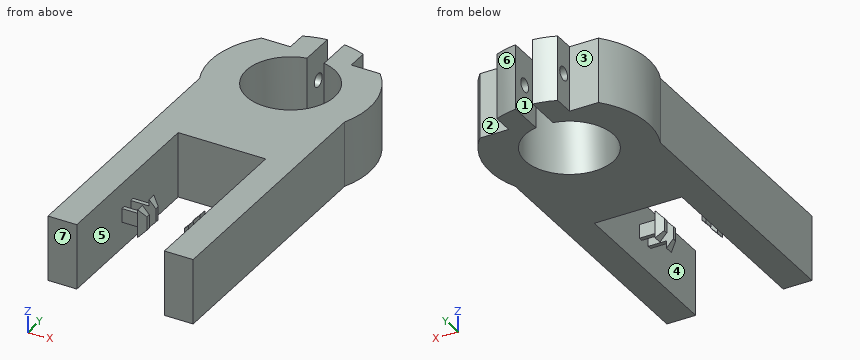
from build123d import *

# Parameters (mm, degrees)
F1_DEPTH = 41.91
F3_DEPTH = 132.842
F4_R     = 4.349558
F5_DEPTH = 93


with BuildPart() as f1:
    # F0 (on Top) → F1 (new body)
    with BuildSketch(Plane.XY):
        with BuildLine():
            ThreePointArc((5.462832, 27.789144), (0, -28.321), (-5.462832, 27.789144))
            Line((-5.462832, 27.789144), (-5.462832, 50.50542))
            ThreePointArc((-5.462832, 50.50542), (-12.596589, 49.213473), (-19.473793, 46.919201))
            Line((-19.473793, 46.919201), (-19.473793, 33.741264))
            Line((-19.473793, 33.741264), (-37.975875, 33.741264))
            ThreePointArc((-37.975875, 33.741264), (-50.191445, 7.839567), (-46.456356, -20.553516))
            Line((-46.456356, -20.553516), (-46.456356, -189.292356))
            Line((-46.456356, -189.292356), (-28.022196, -189.292356))
            Line((-28.022196, -189.292356), (-28.022196, -139.108405))
            Line((-28.022196, -139.108405), (-16.363064, -139.108405))
            Line((-16.363064, -139.108405), (-16.363064, -141.895995))
            Line((-16.363064, -141.895995), (-11.980078, -139.198765))
            Line((-11.980078, -139.198765), (-11.980078, -136.501536))
            Line((-11.980078, -136.501536), (-16.363064, -136.501536))
            Line((-16.363064, -136.501536), (-28.022196, -136.501536))
            Line((-28.022196, -136.501536), (-28.022196, -129.22018))
            Line((-28.022196, -129.22018), (-16.363064, -129.22018))
            Line((-16.363064, -129.22018), (-11.980078, -129.22018))
            Line((-11.980078, -129.22018), (-11.980078, -126.522951))
            Line((-11.980078, -126.522951), (-16.363064, -123.825721))
            Line((-16.363064, -123.825721), (-16.363064, -126.613311))
            Line((-16.363064, -126.613311), (-28.022196, -126.613311))
            Line((-28.022196, -126.613311), (-28.022196, -76.42936))
            Line((-28.022196, -76.42936), (0, -76.42936))
            Line((0, -76.42936), (28.022196, -76.42936))
            Line((28.022196, -76.42936), (28.022196, -126.613311))
            Line((28.022196, -126.613311), (16.363064, -126.613311))
            Line((16.363064, -126.613311), (16.363064, -123.825721))
            Line((16.363064, -123.825721), (11.980078, -126.522951))
            Line((11.980078, -126.522951), (11.980078, -129.22018))
            Line((11.980078, -129.22018), (16.363064, -129.22018))
            Line((16.363064, -129.22018), (28.022196, -129.22018))
            Line((28.022196, -129.22018), (28.022196, -136.501536))
            Line((28.022196, -136.501536), (16.363064, -136.501536))
            Line((16.363064, -136.501536), (11.980078, -136.501536))
            Line((11.980078, -136.501536), (11.980078, -139.198765))
            Line((11.980078, -139.198765), (16.363064, -141.895995))
            Line((16.363064, -141.895995), (16.363064, -139.108405))
            Line((16.363064, -139.108405), (28.022196, -139.108405))
            Line((28.022196, -139.108405), (28.022196, -189.292356))
            Line((28.022196, -189.292356), (46.456356, -189.292356))
            Line((46.456356, -189.292356), (46.456356, -20.553516))
            ThreePointArc((46.456356, -20.553516), (50.191445, 7.839567), (37.975875, 33.741264))
            Line((37.975875, 33.741264), (19.473793, 33.741264))
            Line((19.473793, 33.741264), (19.473793, 46.919201))
            ThreePointArc((19.473793, 46.919201), (12.596589, 49.213473), (5.462832, 50.50542))
            Line((5.462832, 50.50542), (5.462832, 27.789144))
        make_face()
    extrude(amount=F1_DEPTH)

    # F2 (on face) → F3 (cut)
    with BuildSketch(Plane.XZ.offset(76.42936)):
        Polygon((-28.022196, 41.91), (-28.022196, 29.9847), (-28.022196, 25.780085), (-16.324459, 25.780085), (-16.324459, 29.9847), (-11.689119, 24.990531), (12.092193, 24.990531), (16.324459, 29.757692), (16.324459, 25.780085), (28.022196, 25.780085), (28.022196, 29.9847), (28.022196, 41.91), align=None)
        Polygon((-16.324459, 16.899664), (-28.022196, 16.899664), (-28.022196, 11.9253), (-28.022196, 0), (0, 0), (28.022196, 0), (28.022196, 11.9253), (28.022196, 16.899664), (16.324459, 16.899664), (16.324459, 12.152308), (12.092193, 16.919469), (-11.689119, 16.919469), (-16.324459, 11.9253), align=None)
    extrude(amount=F3_DEPTH, mode=Mode.SUBTRACT)

    # F4 (on face) → F5 (cut)
    with BuildSketch(Plane.YZ.offset(19.473793)):
        with Locations((40.330232, 20.955)):
            Circle(F4_R)
    extrude(amount=-F5_DEPTH, mode=Mode.SUBTRACT)


solid = f1.part
The listing builds one solid part. Answer for the finished solid, in the listing's coordinates (mm). Face numbers are marked on the shaded views. A direction names the side the tool comes from. Give positions to 0.01 mm unless a question says otherwise; leave off trailing zeros. Write each loop counter-clockwise with the first axis right and the second up, starting at its lowest first coordinate (ties: lowest second). Pieces come first, ordered by that corner, then holes. Notation, with made-up numbers: (17, 53.5) - (40, 53.5) arc R27 cw to (40, 76.5) - close; hole circle Ø7 at (63.5, 89.5). An arc over 180 degrees is marked (long way). Use a Markdown table: item, result.
1. A tool of negligible diameter and unlimited length cuts with its end or side. For the marked faces 1, 2 and 3, from which of +Z, -Z, +X, -X, +Y, -Y can it reach the whole face along a straight path? Write none if from no direction.
Values follow:
| item | result |
|---|---|
| face 1 | +Z, -Z, +Y |
| face 2 | +Z, -Z, +X, +Y |
| face 3 | +Z, -Z, -X, +Y |
2. Section D-D on y = -50.5 is taken. Write down the section's boundary in (x, z).
Values follow:
| item | result |
|---|---|
| outline | (-46.46, 0) - (46.46, 0) - (46.46, 41.91) - (-46.46, 41.91) - close |
3. Find the intervals of material crossed by probe 1 along X at (y, z) = (-166, 12.5); probe 2 along Y at (x, z) = (-34, 4); probe 3 along Y at (x, z) = (1, 22), in increasing order. Write a range as from..to.
Values follow:
| item | result |
|---|---|
| probe 1 | x = -46.46..-28.02, 28.02..46.46 |
| probe 2 | y = -189.29..33.74 |
| probe 3 | y = -76.43..-28.3 |
4. Section A-A on y = -132 is taken. Write down the section's boundary in (x, z), plus the area to 3 significant figures.
Values follow:
| item | result |
|---|---|
| outline | (-46.46, 0) - (-28.02, 0) - (-28.02, 41.91) - (-46.46, 41.91) - close; (28.02, 0) - (46.46, 0) - (46.46, 41.91) - (28.02, 41.91) - close |
| area | 1,550 mm² |
5. Section C-C on y = 0 is taken. Write down the section's boundary in (x, z).
Values follow:
| item | result |
|---|---|
| outline | (-50.8, 0) - (-28.32, 0) - (-28.32, 41.91) - (-50.8, 41.91) - close; (28.32, 0) - (50.8, 0) - (50.8, 41.91) - (28.32, 41.91) - close |
6. Section B-B on x = 32.5 is taken. Write down the section's boundary in (y, z).
Values follow:
| item | result |
|---|---|
| outline | (-189.29, 0) - (33.74, 0) - (33.74, 41.91) - (-189.29, 41.91) - close |
7. For a pull along X with two mould halves and no side action, classify the marked faces 4, 5, 6 and 7 as released by +X, released by -X, zero draft, split by the parting line, or undercut.
Values follow:
| item | result |
|---|---|
| face 4 | undercut |
| face 5 | undercut |
| face 6 | released by +X |
| face 7 | zero draft |
8. Each of these flat-tipped pins is pushed along its axis until it touches: P1, Ø0.8, axis at y = -127.5, z = 21, coming from the -X side; P2, Ø10, axis at x = 20.5, z = 21, coming from the +Y side; P3, Ø4.5, axis at x = -22.5, y = -139, coming from the -Z side; P4, Ø5, axis at y = 40.33, z = 20.96, coming from the +X side. Where does it stop, or does it pass through?
Values follow:
| item | result |
|---|---|
| P1 | stops at x = -46.46 |
| P2 | stops at y = 48.38 |
| P3 | stops at z = 16.9 |
| P4 | passes through |
